Source: three-view drawing plus pictorial views. Frame: mm from the lowest corner of the part. A direction names the side the tool comes from. Give positions to 0.01 mm unless a question says otherwise; leave off trailing zeros. Loops run counter-clockwise (first coordinate to the right, second up) from the corner with the lowest first, then second, coordinate; pieces in that order, holes last.
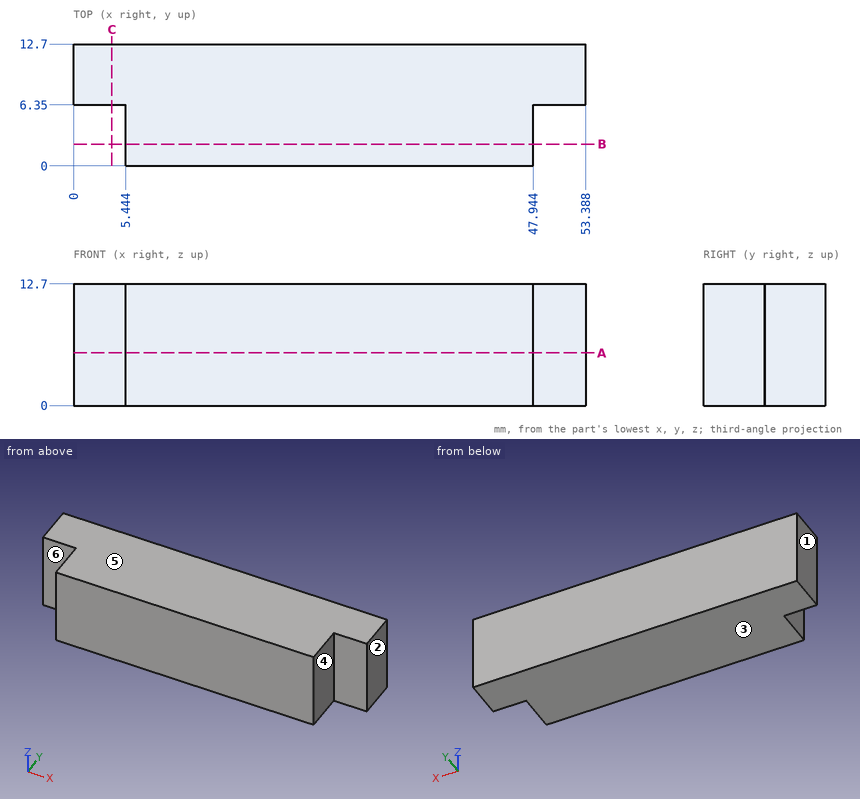
1) Pull-direction query (X, two-part tool) for the marked faces 1, 2 and 3; classes: released by +X, released by -X, zero draft, split by the parting line, or undercut.
Checks:
face 1: released by -X
face 2: released by +X
face 3: zero draft
2) Reachability of the marked faces 4, 5 and 6 from +Z, -Z, +X, -X, +Y, -Y: full face, straight path, thin tool, end or side. Return the list, or none.
Checks:
face 4: +Z, -Z, +X, -Y
face 5: +Z, +X, -X, +Y, -Y
face 6: +Z, -Z, -X, -Y
3) Cut plane A-A (z = 5.5). Return loops of the section in (x, y).
Checks:
outline: (0, 6.35) - (5.44, 6.35) - (5.44, 0) - (47.94, 0) - (47.94, 6.35) - (53.39, 6.35) - (53.39, 12.7) - (0, 12.7) - close
4) Cut plane C-C (x = 4). Return loops of the section in (y, z).
Checks:
outline: (6.35, 0) - (12.7, 0) - (12.7, 12.7) - (6.35, 12.7) - close
5) Ray query, probe 1 along X at (y, z) = (2.5, 11.5). Return the intervals inside material, ascending.
Checks:
probe 1: x = 5.44 to 47.94
6) Cut plane B-B (y = 2.25). Return loops of the section in (x, z), and give its area (3 significant figures).
Checks:
outline: (5.44, 0) - (47.94, 0) - (47.94, 12.7) - (5.44, 12.7) - close
area: 540 mm2
7) Contact query for flat-ended pins moving along their axis: P1, Ø1, axis at x = 6, z = 1.5, coming from the -Y side; P2, Ø7, axis at y = 2.5, z = 7, coming from the -X side; P3, Ø3, axis at y = 4.5, z = 4.5, coming from the +X side; P4, Ø2.5, axis at x = 2, z = 8.5, coming from the -Y side. Output: stop coordinate, or through.
Checks:
P1: stops at y = 0
P2: stops at x = 5.44
P3: stops at x = 47.94
P4: stops at y = 6.35
